Study the drawing (mm; zero at the part's minimum x, y, z) and answer. Give positions to 0.01 mm unless a question says otherwise; leave off trailing zeros. Order: outer loops, then holes, each group sorted by start corner. A loop starts at its lowest first (then second) coordinate and runs counter-clockwise, first axis right, second up.
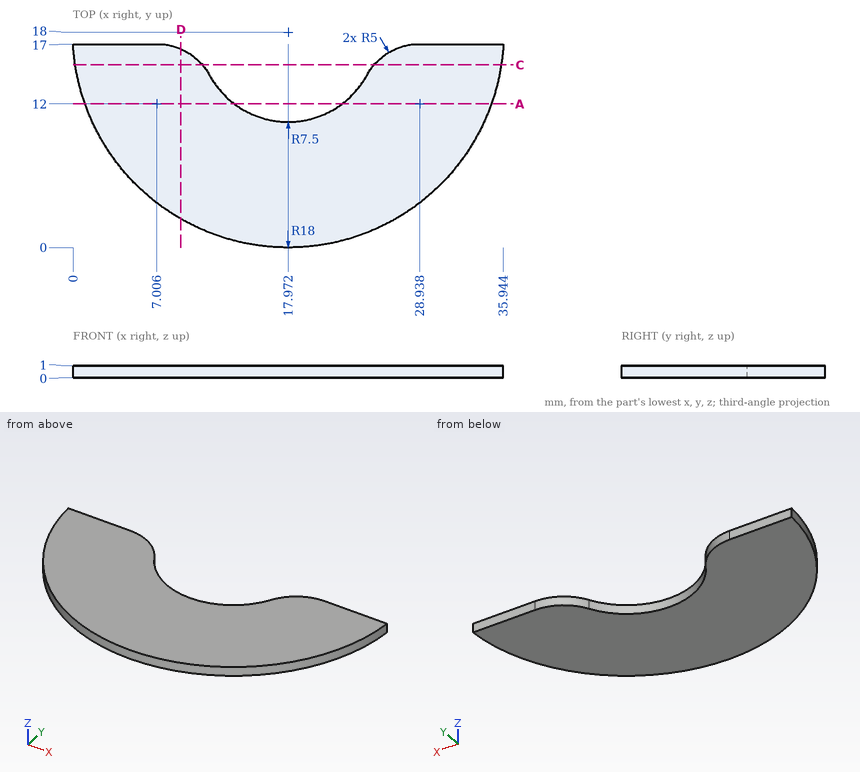
1) Find section C-C (y = 15.25). Write down the section's boundary in (x, z).
Geometry says:
outline: (0.18, 0) - (10.81, 0) - (10.81, 1) - (0.18, 1) - close; (25.14, 0) - (35.76, 0) - (35.76, 1) - (25.14, 1) - close
2) Find section A-A (y = 12). Write down the section's boundary in (x, z).
Geometry says:
outline: (1, 0) - (13.47, 0) - (13.47, 1) - (1, 1) - close; (22.47, 0) - (34.94, 0) - (34.94, 1) - (22.47, 1) - close
3) Straight lines are drawn through the part: probe 1 along X at (y, z) = (12.5, 0.8) (1 decimal); probe 2 along X at (y, z) = (15, 0.1) (1 decimal); probe 3 along X at (y, z) = (7.5, 0.6). For each, find the intervals that lie inside material, in ascending order.
Geometry says:
probe 1: x = 0.8 to 12.9, 23.1 to 35.1
probe 2: x = 0.2 to 11, 24.9 to 35.7
probe 3: x = 3.35 to 32.59
4) Find section D-D (x = 9). Write down the section's boundary in (y, z) (1 decimal), then the cut area to 3 significant figures.
Geometry says:
outline: (2.4, 0) - (16.6, 0) - (16.6, 1) - (2.4, 1) - close
area: 14.2 mm2
